Autodesk Inventor part; units mm, degrees
ref_plane "YZ Plane" through (0, 0, 0) normal (1, 0, 0) x (0, 1, 0)
ref_plane "XZ Plane" through (0, 0, 0) normal (0, 1, 0) x (-1, 0, 0)
ref_plane "XY Plane" through (0, 0, 0) normal (0, 0, 1) x (1, 0, 0)
sketch "Skizze1" plane through (0, 0, 0) normal (0, 0, 1) x (1, 0, 0)
  line L0 (-27.95, 27.95) -> (27.95, 27.95)
  line L1 (27.95, 27.95) -> (27.95, -27.95)
  line L2 (27.95, -27.95) -> (-27.95, -27.95)
  line L3 (-27.95, -27.95) -> (-27.95, 27.95)
  line L4 (-27.95, 27.95) -> (27.95, -27.95) construction
  line L5 (27.95, 27.95) -> (-27.95, -27.95) construction
  point P0 (0, 0)
  dimension "d0" = 55.9
  dimension "d1" = 55.9
extrude "Extrusion1" add sketch "Skizze1" along normal blind 2
sketch "Skizze2" plane through (0, 0, 2) normal (0, 0, 1) x (1, 0, 0)
  line L0 (-27.95, -27.95) -> (27.95, -27.95)
  line L1 (27.95, -27.95) -> (27.95, 27.95)
  line L2 (27.95, 27.95) -> (-27.95, 27.95)
  line L3 (-27.95, 27.95) -> (-27.95, -27.95)
  line L4 (-25.95, 25.95) -> (25.95, 25.95)
  line L5 (25.95, 25.95) -> (25.95, -25.95)
  line L6 (25.95, -25.95) -> (-25.95, -25.95)
  line L7 (-25.95, -25.95) -> (-25.95, 25.95)
  point P0 (0, 0)
  dimension "d4" = 2
extrude "Extrusion2" add sketch "Skizze2" along normal blind 5
fillet "Rundung1" radius 2 4 edges at (-27.95, -27.95, 3.5) (27.95, -27.95, 3.5) (27.95, 27.95, 3.5) (-27.95, 27.95, 3.5)
sketch "Skizze5" plane through (0, 0, 2) normal (0, 0, 1) x (1, 0, 0)
  line L0 (-23.5, 10) -> (23.5, 10) construction
  line L1 (23.5, 10) -> (23.5, -10) construction
  line L2 (23.5, -10) -> (-23.5, -10) construction
  line L3 (-23.5, -10) -> (-23.5, 10) construction
  line L4 (-23.5, 10) -> (23.5, -10) construction
  line L5 (23.5, 10) -> (-23.5, -10) construction
  arc A0 (-23.5, -13.5) -> (-23.5, -6.5) centre (-23.5, -10) ccw
  arc A1 (-23.5, 6.5) -> (-23.5, 13.5) centre (-23.5, 10) ccw
  arc A2 (23.5, 13.5) -> (23.5, 6.5) centre (23.5, 10) ccw
  arc A3 (23.5, -6.5) -> (23.5, -13.5) centre (23.5, -10) ccw
  line L6 (-25.95, 25.95) -> (25.95, 25.95)
  line L7 (-25.95, -25.95) -> (-25.95, 25.95)
  line L8 (25.95, -25.95) -> (-25.95, -25.95)
  line L9 (25.95, 25.95) -> (25.95, -25.95)
  line L10 (23.5, -13.5) -> (25.95, -13.5)
  line L11 (23.5, -6.5) -> (25.95, -6.5)
  line L12 (23.5, 6.5) -> (25.95, 6.5)
  line L13 (23.5, 13.5) -> (25.95, 13.5)
  line L14 (-23.5, 13.5) -> (-25.95, 13.5)
  line L15 (-23.5, 6.5) -> (-25.95, 6.5)
  line L16 (-23.5, -6.5) -> (-25.95, -6.5)
  line L17 (-23.5, -13.5) -> (-25.95, -13.5)
  point P0 (0, 0)
  point P1 (-23.95, 25.95)
  point P2 (23.95, 25.95)
  point P3 (-25.95, -23.95)
  point P4 (-25.95, 23.95)
  point P5 (23.95, -25.95)
  point P6 (-23.95, -25.95)
  point P7 (25.95, 23.95)
  point P8 (25.95, -23.95)
  dimension "d17" = 47
  dimension "d18" = 20
  dimension "d19" = 7
  dimension "d20" = 7
  dimension "d21" = 7
  dimension "d22" = 7
extrude "Extrusion3" add sketch "Skizze5" along normal blind 5 contours L17 L7 L16 A0 | L7 L14 A1 L15 | L10 A3 L11 L9 | L12 A2 L13 L9
sketch "Skizze3" plane through (0, 0, 0) normal (0, 0, -1) x (-1, 0, 0)
  line L0 (23.5, 10) -> (-23.5, 10)
  line L1 (-23.5, 10) -> (-23.5, -10)
  line L2 (-23.5, -10) -> (23.5, -10)
  line L3 (23.5, -10) -> (23.5, 10)
  line L4 (23.5, 10) -> (-23.5, -10) construction
  line L5 (-23.5, 10) -> (23.5, -10) construction
  point P0 (0, 0)
  dimension "d8" = 47
  dimension "d9" = 20
hole "Bohrung1" at (23.5, -10, 0) at (23.5, 10, 0) at (-23.5, 10, 0) at (-23.5, -10, 0) direction (0, 0, 1) diameter 3 end through all counterbore diameter 6 counterbore depth 2
chamfer "Fasen1" distance 0.5 angle 45 12 edges at (0, -27.95, 0) (27.3642, -27.3642, 0) (27.95, 0, 0) (27.3642, 27.3642, 0) (0, 27.95, 0) (-27.3642, 27.3642, 0) (-27.95, 0, 0) (-27.3642, -27.3642, 0) (-23.5, -13, 0) (23.5, -13, 0) (-23.5, 7, 0) (23.5, 7, 0)
properties part number "BlindCover"
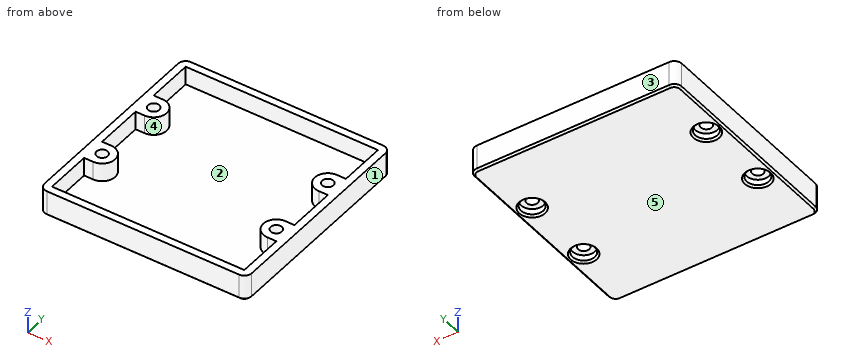
Check sheet for the modelled part. Datum: model origin and axes. Units: mm. Face numbers are marked on the shaded views. A direction names the side the tool comes from. Give positions to 0.01 mm unless a question says otherwise; leave off trailing zeros. Write each loop counter-clockwise with the first axis right and the second up, starting at its lowest first coordinate (ties: lowest second). Pieces come first, ordered by that corner, then holes. Notation, with made-up numbers: (-26.5, 69.25) -> (6.5, 69.25) arc R21 ccw to (6.5, 107.25) -> close; hole circle Ø6 at (69.25, -33). An arc over 180 degrees is marked (long way). Use one line per item in the form item = value. Start each with the question number.
1. Thickness scan on line 1 along Y through (x, z) = (23.5, 1.1); line 2 along Y through (x, z) = (23.5, 5.05); line 3 along X through (y, z) = (10, 4.7). Record the ranges inside material, lowest first. Write a range as from..to.
2. Section check A-A (y = 10). Count the separate pieces of the cut face and the enclosed holes in it, and give its area (3 significant figures).
3. Section check C-C (y = 20.5). Record the cut outline in (x, z), and give its area (3 significant figures).
4. Access from +Z, -Z, +X, -X, +Y, -Y to the whole of each face (thin tool, end or side, straight path). Record for the marked faces 1 and 2.
5. Go/stop test with flat-tipped pins: P1, Ø3.5, axis at x = 23.5, y = -10, coming from the -Z side; P2, Ø1, axis at x = 14, y = 4, coming from the +Z side. Record where each tip stops, or that it passes through.
6. Mould release check, pull along Y, two halves, no side actions. Record for the marked faces 3, 4 and 5: pulls with the +Y half, pulls with the -Y half, needs draft (parallel to the pull), parting line crosses it, or undercut.
Conclusion:
q1.line_1 = -27.95..-13, -7..7, 13..27.95
q1.line_2 = -27.95..-25.95, -13.5..-11.5, -8.5..-6.5, 6.5..8.5, 11.5..13.5, 25.95..27.95
q1.line_3 = -27.95..-25, -22..-20, 20..22, 25..27.95
q2.separate_pieces = 3
q2.enclosed_holes = 0
q2.area = 137 mm²
q3.outline = (-27.95, 0.5) -> (-27.45, 0) -> (27.45, 0) -> (27.95, 0.5) -> (27.95, 7) -> (25.95, 7) -> (25.95, 2) -> (-25.95, 2) -> (-25.95, 7) -> (-27.95, 7) -> close
q3.area = 132 mm²
q4.face_1 = +Z, -Z, +X, +Y, -Y
q4.face_2 = +Z
q5.P1 = 2
q5.P2 = 2
q6.face_3 = pulls with the +Y half
q6.face_4 = undercut
q6.face_5 = needs draft
